```python
from build123d import *

# Parameters (mm, degrees)
CROQUIS1_W              = 111
CROQUIS1_H              = 64
CROQUIS1_R              = 1.6
SALIENTE_EXTRUIR1_DEPTH = 5
CROQUIS2_W              = 5
CROQUIS2_H              = 21.3333333
SALIENTE_EXTRUIR2_DEPTH = 5
CROQUIS3_W              = 5
CROQUIS3_H              = 21.3333333
SALIENTE_EXTRUIR3_DEPTH = 5


with BuildPart() as part:
    # Croquis1 → Saliente-Extruir1 (new body)
    with BuildSketch(Plane.XY):
        with Locations((13.812375919, -5.640074375)):
            Rectangle(CROQUIS1_W, CROQUIS1_H)
        with Locations((-20.317624082, -30.440068587)):
            Circle(CROQUIS1_R, mode=Mode.SUBTRACT)
        with Locations((-19.047624082, 17.819931413)):
            Circle(CROQUIS1_R, mode=Mode.SUBTRACT)
        with Locations((55.882375918, 17.819931413)):
            Circle(CROQUIS1_R, mode=Mode.SUBTRACT)
        with Locations((62.232375918, -30.440068587)):
            Circle(CROQUIS1_R, mode=Mode.SUBTRACT)
        with BuildLine():
            Line((-27.547897963, 14.398218547), (57.441208347, 14.398218547))
            ThreePointArc((57.441208347, 14.398218547), (58.7657139, 13.073712995), (57.441208347, 11.749207442))
            Line((57.441208347, 11.749207442), (-27.547897963, 11.749207442))
            ThreePointArc((-27.547897963, 11.749207442), (-28.872403516, 13.073712995), (-27.547897963, 14.398218547))
        make_face(mode=Mode.SUBTRACT)
        with BuildLine():
            Line((-27.547897963, 8.398218547), (57.441208347, 8.398218547))
            ThreePointArc((57.441208347, 8.398218547), (58.7657139, 7.073712995), (57.441208347, 5.749207442))
            Line((57.441208347, 5.749207442), (-27.547897963, 5.749207442))
            ThreePointArc((-27.547897963, 5.749207442), (-28.872403516, 7.073712995), (-27.547897963, 8.398218547))
        make_face(mode=Mode.SUBTRACT)
        with BuildLine():
            Line((-27.547897963, 2.398218547), (57.441208347, 2.398218547))
            ThreePointArc((57.441208347, 2.398218547), (58.7657139, 1.073712995), (57.441208347, -0.250792558))
            Line((57.441208347, -0.250792558), (-27.547897963, -0.250792558))
            ThreePointArc((-27.547897963, -0.250792558), (-28.872403516, 1.073712995), (-27.547897963, 2.398218547))
        make_face(mode=Mode.SUBTRACT)
        with BuildLine():
            Line((-27.547897963, -3.601781453), (57.441208347, -3.601781453))
            ThreePointArc((57.441208347, -3.601781453), (58.7657139, -4.926287005), (57.441208347, -6.250792558))
            Line((57.441208347, -6.250792558), (-27.547897963, -6.250792558))
            ThreePointArc((-27.547897963, -6.250792558), (-28.872403516, -4.926287005), (-27.547897963, -3.601781453))
        make_face(mode=Mode.SUBTRACT)
        with BuildLine():
            Line((-27.547897963, -9.601781453), (57.441208347, -9.601781453))
            ThreePointArc((57.441208347, -9.601781453), (58.7657139, -10.926287005), (57.441208347, -12.250792558))
            Line((57.441208347, -12.250792558), (-27.547897963, -12.250792558))
            ThreePointArc((-27.547897963, -12.250792558), (-28.872403516, -10.926287005), (-27.547897963, -9.601781453))
        make_face(mode=Mode.SUBTRACT)
        with BuildLine():
            Line((-27.547897963, -15.601781453), (57.441208347, -15.601781453))
            ThreePointArc((57.441208347, -15.601781453), (58.7657139, -16.926287005), (57.441208347, -18.250792558))
            Line((57.441208347, -18.250792558), (-27.547897963, -18.250792558))
            ThreePointArc((-27.547897963, -18.250792558), (-28.872403516, -16.926287005), (-27.547897963, -15.601781453))
        make_face(mode=Mode.SUBTRACT)
        with BuildLine():
            Line((-27.547897963, -21.601781453), (57.441208347, -21.601781453))
            ThreePointArc((57.441208347, -21.601781453), (58.7657139, -22.926287005), (57.441208347, -24.250792558))
            Line((57.441208347, -24.250792558), (-27.547897963, -24.250792558))
            ThreePointArc((-27.547897963, -24.250792558), (-28.872403516, -22.926287005), (-27.547897963, -21.601781453))
        make_face(mode=Mode.SUBTRACT)
    extrude(amount=SALIENTE_EXTRUIR1_DEPTH)

    # Croquis2 → Saliente-Extruir2 (add)
    with BuildSketch(Plane.ZY.offset(41.687624081)):
        with Locations((2.5, -5.640074358)):
            Rectangle(CROQUIS2_W, CROQUIS2_H)
    extrude(amount=SALIENTE_EXTRUIR2_DEPTH)

    # Croquis3 → Saliente-Extruir3 (add)
    with BuildSketch(Plane(origin=(69.312375919, 0, 0), x_dir=(0, 0, -1), z_dir=(1, 0, 0))):
        with Locations((-2.5, -5.640074358)):
            Rectangle(CROQUIS3_W, CROQUIS3_H)
    extrude(amount=SALIENTE_EXTRUIR3_DEPTH)


solid = part.part
```
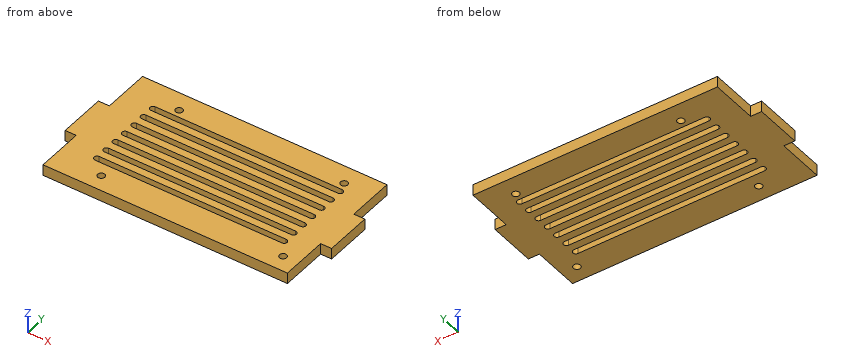
Input: part model. Units: mm. Frame: model coordinates. Coordinates: 2 decimals unless noted, no trailing zeros. Write each question's results on one line, items separated by ' | '.
Item 1: Pin query (flat end, axial travel): pin 1 Ø1.5 at (y, z) = (18, 3) entering from -X; pin 2 Ø1.9 at (x, y) = (55.88, 17.82) entering from -Z. Return the tip coordinate at first contact, or that it passes through.
Conclusion:
pin 1: stops at x = -41.69 | pin 2: passes through
Item 2: Material intervals for probe 1 along X at (y, z) = (16.5, 2.7); probe 2 along X at (y, z) = (-17, 4.85); probe 3 along X at (y, z) = (-11, 4.5), sorted ascending.
Conclusion:
probe 1: x = -41.69 to -19.95, -18.14 to 54.98, 56.79 to 69.31 | probe 2: x = -41.69 to -28.87, 58.76 to 69.31 | probe 3: x = -46.69 to -28.87, 58.76 to 74.31
Item 3: Section query A-A on x = -10.5. Count the separate pieces of the cut face and the enclosed holes in it, plus the area to 3 significant figures.
Conclusion:
separate pieces: 8 | enclosed holes: 0 | area: 227 mm^2
